from build123d import *

# Parameters (mm, degrees)
F0_W     = 8.562588
F0_H     = 9
F1_DEPTH = 58
F3_DEPTH = 11
F4_R     = 3
F6_DEPTH = 38.001


with BuildPart() as f1:
    # F0 (on Front) → F1 (new body)
    with BuildSketch(Plane.XZ):
        with BuildLine():
            Line((-49.456521, 9), (-49.456521, 0))
            Line((-49.456521, 0), (55.543479, 0))
            Line((55.543479, 0), (55.543479, 9))
            Line((55.543479, 9), (66.543479, 9))
            ThreePointArc((66.543479, 9), (58.049576, 29.506097), (37.543479, 38))
            Line((37.543479, 38), (-40.019109, 38))
            ThreePointArc((-40.019109, 38), (-60.525206, 29.506097), (-69.019109, 9))
            Line((-69.019109, 9), (-58.019109, 9))
            Line((-58.019109, 9), (-49.456521, 9))
        make_face()
        with Locations((-53.737815, 4.5)):
            Rectangle(F0_W, F0_H)
    extrude(amount=-F1_DEPTH)

    # F2 (on face) → F3 (cut)
    with BuildSketch(Plane.XY.offset(38)):
        Polygon((-64.201698, 11), (0, 11), (60.26233, 11), (64.404465, 11), (64.404465, 47), (60.26233, 47), (0, 47), (-64.201698, 47), align=None)
    extrude(amount=-F3_DEPTH, mode=Mode.SUBTRACT)

    # F4
    f4_edges = [f1.edges().sort_by_distance(p)[0] for p in [
        (-1.237815, 0, 38),
        (-1.237815, 58, 38),
        (-60.525206, 0, 29.506097),
        (58.049576, 0, 29.506097),
        (-60.525206, 58, 29.506097),
        (58.049576, 58, 29.506097),
    ]]
    fillet(f4_edges, radius=F4_R)

    # F5 (on face) → F6 (cut, through all)
    with BuildSketch(Plane(origin=(0, 0, 0), x_dir=(1, 0, 0), z_dir=(0, 0, -1))):
        with BuildLine():
            Line((-25.019109, -22.5), (-44.019109, -22.5))
            ThreePointArc((-44.019109, -22.5), (-48.615303, -24.403806), (-50.519109, -29))
            ThreePointArc((-50.519109, -29), (-48.615303, -33.596194), (-44.019109, -35.5))
            Line((-44.019109, -35.5), (-25.019109, -35.5))
            ThreePointArc((-25.019109, -35.5), (-18.519109, -29), (-25.019109, -22.5))
        make_face()
        with BuildLine():
            Line((41.543479, -22.5), (22.543479, -22.5))
            ThreePointArc((22.543479, -22.5), (16.043479, -29), (22.543479, -35.5))
            Line((22.543479, -35.5), (41.543479, -35.5))
            ThreePointArc((41.543479, -35.5), (46.139673, -33.596194), (48.043479, -29))
            ThreePointArc((48.043479, -29), (46.139673, -24.403806), (41.543479, -22.5))
        make_face()
    extrude(amount=-F6_DEPTH, mode=Mode.SUBTRACT)


solid = f1.part
The listing builds one solid part. Answer for the finished solid, in the listing's coordinates (mm). A direction names the side the tool comes from. Round coordinates to 2 decimals unless told otherwise and drop trailing zeros. Loops run counter-clockwise (first coordinate to the right, second up) from the corner with the lowest first, then second, coordinate; pieces in that order, holes last. Notation, with made-up numbers: M 66,-20 L 99,-20 A24 cw 99,-4 Z; hole C 80,48.5 d10. An arc over 180 degrees is marked long. Write each question's results on one line, items separated by ' | '. Start each with the question number.
1) Find section B-B on y = 33. Write down the section's boundary in (x, z).
2) Find section D-D on y = 21. Write down the section's boundary in (x, z), plus the area to 3 significant figures.
3) Straight lines are drawn through the part: probe 1 along Y at (x, z) = (23, 13.5); probe 2 along Y at (x, z) = (32.5, 30.5); probe 3 along Z at (x, y) = (-15, 33). For each, find the intervals that lie inside material, in ascending order.
4) Find section A-A on z = 7. Write down the section's boundary in (x, y), plus the area to 3 significant figures.
5) Find section C-C on x = 0.5. Write down the section's boundary in (y, z), plus the area to 3 significant figures.
6) Each of these flat-tipped pins is pushed along its axis until it touches: pin 1 (2.5 mm diameter, centred on y = 20, z = 6, fed in from +X); pin 2 (12 mm diameter, centred on x = 18, y = 27.5, fed in from +Z); pin 3 (3.5 mm diameter, centred on x = -64, y = 23.5, fed in from -Z). Where does it stop, or does it pass through?
7) Which of the six approach directions +Z, -Z, +X, -X, +Y, -Y give full straight-line access (tool end or side, diameter ignored) to faces 1 (the flat face through (-2, 11, 33)), 2 (the flat face through (-58.019, 29, 4)), 3 (the flat face through (61, 29, 9)), 4 (the flat face through (-2, 29, 0)), 5 (the flat face through (-35, 35.5, 13))?
8) Determine the mould class of faces 6 (the flat face through (-2, 58, 18)), 7 (the flat face through (-1, 7, 38)), 8 (the cylindrical face through (16.045, 28.857, 13.311)) for opening direction Y: pulls with the +Y half, pulls with the -Y half, needs draft (parallel to the pull), parting line crosses it, or undercut.
Final values:
1) outline: M -69.02,9 L -58.02,9 L -58.02,0 L -49.14,0 L -49.14,27 L -62.76,27 A29 ccw Z; M -19.9,0 L 17.42,0 L 17.42,27 L -19.9,27 Z; M 46.67,0 L 55.54,0 L 55.54,9 L 66.54,9 A29 ccw 60.28,27 L 46.67,27 Z
2) outline: M -69.02,9 L -58.02,9 L -58.02,0 L 55.54,0 L 55.54,9 L 66.54,9 A29 ccw 60.28,27 L -62.76,27 A29 ccw Z | area: 3,390 mm²
3) probe 1: 0 to 22.5, 35.5 to 58 | probe 2: 0 to 11, 47 to 58 | probe 3: 0 to 27
4) outline: M -58.02,0 L 55.54,0 L 55.54,58 L -58.02,58 Z; hole M -44.02,22.5 L -25.02,22.5 A6.5 ccw -25.02,35.5 L -44.02,35.5 A6.5 ccw Z; hole M 22.54,22.5 L 41.54,22.5 A6.5 ccw 41.54,35.5 L 22.54,35.5 A6.5 ccw Z | area: 5,830 mm²
5) outline: M 0,0 L 58,0 L 58,35 A3 ccw 55,38 L 47,38 L 47,27 L 11,27 L 11,38 L 3,38 A3 ccw 0,35 Z | area: 1,800 mm²
6) pin 1: x = 55.54 | pin 2: z = 27 | pin 3: z = 9
7) face 1: +Z, +X, -X | face 2: -Z, -X, +Y, -Y | face 3: -Z, +X, +Y, -Y | face 4: -Z, +X, -X, +Y, -Y | face 5: +Z, -Z
8) face 6: pulls with the +Y half | face 7: needs draft | face 8: undercut
